Part print with two shaded views. Sizes in mm from the minimum x, y, z corner. Give positions to 0.01 mm unless a question says otherwise; leave off trailing zeros. Write each loop counter-clockwise with the first axis right and the second up, starting at its lowest first coordinate (ties: lowest second). Pieces come first, ordered by that corner, then holes. Notation, with made-up numbers: (-7.5, -17.5) -> (49.5, -17.5) arc R16 cw to (49.5, 3.5) -> close; hole circle Ø6 at (69, 59.5). An arc over 180 degrees is marked (long way). Answer as a JSON object with one key per item and string values.
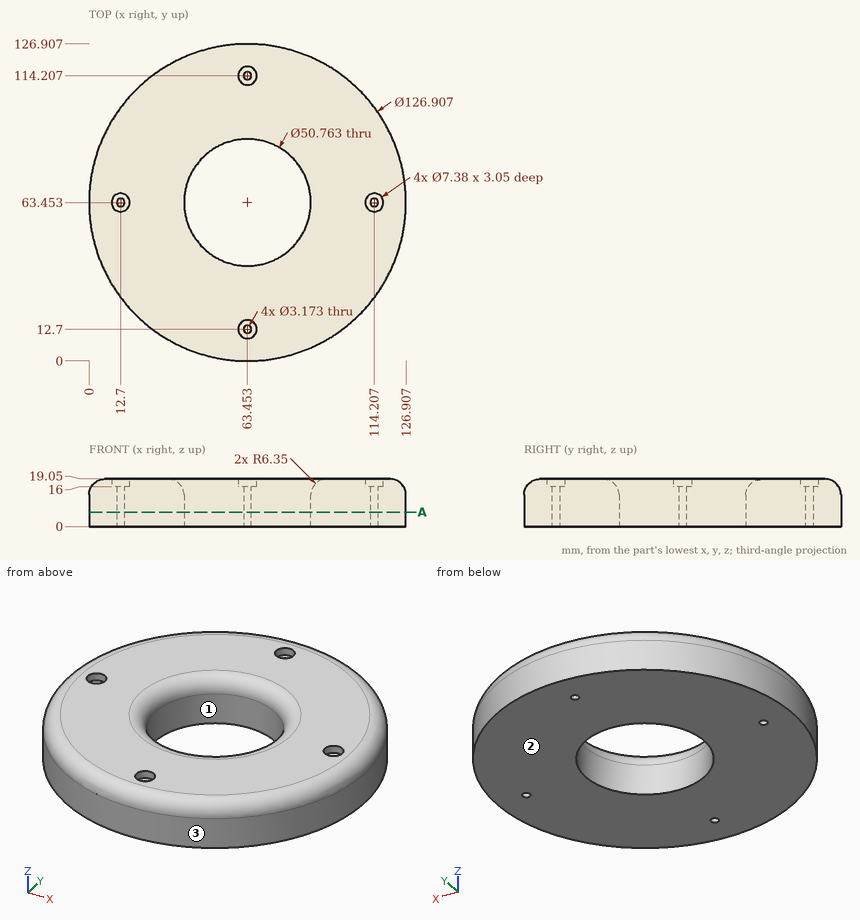
1) Pin check, flat tips, straight feed: pin 1 (4 mm diameter, centred on x = 12.7, y = 63.45, fed in from +Z); pin 2 (10 mm diameter, centred on x = 51, z = 7, fed in from -Y); pin 3 (6 mm diameter, centred on x = 23.5, z = 16, fed in from -Y); pin 4 (2.5 mm diameter, centred on x = 63.45, y = 12.7, fed in from -Z). Stop position of each tip, or through.
Model answer:
{"pin 1": "stops at z = 16", "pin 2": "stops at y = 0.44", "pin 3": "stops at y = 12.48", "pin 4": "passes through"}
2) Mould opens along Y. For the marked faces 1, 2 and 3 say: released by +Y, released by -Y, zero draft, split by the parting line, or undercut.
Model answer:
{"face 1": "undercut", "face 2": "zero draft", "face 3": "split by the parting line"}
3) Slice it at A-A (z = 5.75). List the corners of the cut face in (x, y) (1 decimal).
Model answer:
{"outline": "circle Ø126.9 at (63.5, 63.5); hole circle Ø3.2 at (12.7, 63.5); hole circle Ø50.8 at (63.5, 63.5); hole circle Ø3.2 at (63.5, 12.7); hole circle Ø3.2 at (63.5, 114.2); hole circle Ø3.2 at (114.2, 63.5)"}
4) Wall check: probe 1 along Y at (x, z) = (86, 11) (1 decimal); probe 2 along X at (y, z) = (87, 15.25) (1 decimal); probe 3 along X at (y, z) = (41, 6.75) (1 decimal). Give the ranges that are in metal, low to high.
Model answer:
{"probe 1": "y = 4.1 to 51.8, 75.1 to 122.8", "probe 2": "x = 5.1 to 52.6, 74.3 to 121.8", "probe 3": "x = 4.1 to 51.6, 75.3 to 122.8"}
